from build123d import *

# Parameters (mm, degrees)
SKETCH_R      = 37.35
PAD_DEPTH     = 23.6
THICKNESS_T   = -1.6
SKETCH001_R   = 37.35
SKETCH001_R_2 = 29
PAD001_DEPTH  = 1.6
SKETCH002_W   = 71.5
SKETCH002_H   = 22
POCKET_DEPTH  = 50


with BuildPart() as part:
    # Sketch → Pad (new body)
    with BuildSketch(Plane.XY):
        Circle(SKETCH_R)
    extrude(amount=PAD_DEPTH)

    # Thickness
    thickness_openings = [part.faces().sort_by_distance(p)[0] for p in [
        (0, 0, 23.6),
    ]]
    offset(amount=THICKNESS_T, openings=thickness_openings)

    # Sketch001 (on Face3 of Thickness) → Pad001 (join)
    with BuildSketch(Plane.XY.offset(23.6)):
        Circle(SKETCH001_R)
        Circle(SKETCH001_R_2, mode=Mode.SUBTRACT)
    extrude(amount=PAD001_DEPTH)

    # Sketch002 → Pocket (cut)
    with BuildSketch(Plane.XZ):
        with Locations((0, 12.6)):
            Rectangle(SKETCH002_W, SKETCH002_H)
    extrude(amount=-POCKET_DEPTH, mode=Mode.SUBTRACT)


solid = part.part
Can you work these out from the model? Positions are in its coordinate system, mm. A direction names the side the tool comes from. Round coordinates to 2 decimals unless told otherwise and drop trailing zeros. Order: outer loops, then holes, each group sorted by start corner. A loop starts at its lowest first (then second) coordinate and runs counter-clockwise, first axis right, second up. Notation, with made-up numbers: M -29,76.25 L 20,76.25 A17 ccw 20,84.25 Z; hole C -27.75,-26 d5. An arc over 180 degrees is marked long. Use a Markdown table: item, result.
1) If we mould it in two halves opening along Z, with no side actions, what happens to faces 3 (the face through (-11, 28, 23.6)), 4 (the face through (-1, 1, 0)), 5 (the face through (13.38, -25.73, 24.39)), 6 (the face through (19.2, -22, 25.2))? For each: +Z half, -Z half, draft (parallel to the pull), parting line (faces both ways), or undercut.
Geometry says:
| item | result |
|---|---|
| face 3 | undercut |
| face 4 | -Z half |
| face 5 | draft |
| face 6 | +Z half |
2) Imagine slicing it at C-C (x = -10). List the corners of the cut face in (y, z) for me, then the cut area to 3 significant figures.
Geometry says:
| item | result |
|---|---|
| outline | M -35.99,0 L 35.99,0 L 35.99,1.6 L -34.32,1.6 L -34.32,23.6 L -27.22,23.6 L -27.22,25.2 L -35.99,25.2 Z; M 27.22,23.6 L 35.99,23.6 L 35.99,25.2 L 27.22,25.2 Z |
| area | 180 mm² |
3) Imagine slicing it at B-B (y = 15.5). List the corners of the cut face in (x, z) for me.
Geometry says:
| item | result |
|---|---|
| outline | M -33.98,0 L 33.98,0 L 33.98,1.6 L -33.98,1.6 Z; M -33.98,23.6 L -24.51,23.6 L -24.51,25.2 L -33.98,25.2 Z; M 24.51,23.6 L 33.98,23.6 L 33.98,25.2 L 24.51,25.2 Z |
4) If I drill on line 1 along Y through (x, z) = (0, 24.75); line 2 along Z through (x, y) = (0, -32.5); line 3 along Z through (x, y) = (10, -18), over which ranges is the centre line in solid material (lowest first)?
Geometry says:
| item | result |
|---|---|
| line 1 | y = -37.35 to -29, 29 to 37.35 |
| line 2 | z = 0 to 1.6, 23.6 to 25.2 |
| line 3 | z = 0 to 1.6 |
5) Imagine slicing it at D-D (y = 3.5). List the corners of the cut face in (x, z) for me, then the cut area to 3 significant figures.
Geometry says:
| item | result |
|---|---|
| outline | M -37.19,0 L 37.19,0 L 37.19,25.2 L 28.79,25.2 L 28.79,23.6 L 35.75,23.6 L 35.75,1.6 L -35.75,1.6 L -35.75,23.6 L -28.79,23.6 L -28.79,25.2 L -37.19,25.2 Z |
| area | 209 mm² |
6) On a 3-axis mill with a long thin cutter (end or side, diameter ignored), from which of +Z, -Z, +X, -X, +Y, -Y can I reach the whole of each face in a straight line? I mean faces 1 (the face through (-8.1, -36.46, 12.42)), 2 (the face through (-1, 0, 1.6)). Say none if no direction works.
Geometry says:
| item | result |
|---|---|
| face 1 | +Z, -Z |
| face 2 | +Y |
7) I'm going to push flat-ended pins straight in: P1, Ø6, axis at x = 1.5, z = 4, coming from the +Y side; P2, Ø1, axis at x = -16, y = -23, coming from the +Z side; P3, Ø12, axis at x = 24, z = 12, coming from the +Y side; P4, Ø5.5, axis at y = 5.5, z = 8, coming from the -X side. Where does each tip first touch, or does it pass through?
Geometry says:
| item | result |
|---|---|
| P1 | stops at y = 37.35 |
| P2 | stops at z = 1.6 |
| P3 | stops at y = -19.44 |
| P4 | stops at x = -37.25 |
8) Imagine slicing it at A-A (x = 0). List the corners of the cut face in (y, z) for me.
Geometry says:
| item | result |
|---|---|
| outline | M -37.35,0 L 37.35,0 L 37.35,1.6 L -35.75,1.6 L -35.75,23.6 L -29,23.6 L -29,25.2 L -37.35,25.2 Z; M 29,23.6 L 37.35,23.6 L 37.35,25.2 L 29,25.2 Z |
